Can you work these out from the model? Positions are in its coordinate system, mm. A direction names the side the tool comes from. Round coordinates to 2 decimals unless told otherwise and drop trailing zeros. Order: outer loops, then holes, each group sorted by start corner. A loop starts at its lowest first (then second) coordinate and runs counter-clockwise, first axis right, second up. Notation, with made-up numbers: (-25.75, -7.75) -> (26.25, -7.75) arc R19 cw to (26.25, -1.75) -> close; hole circle Ø5 at (52, 70.25). An arc over 180 degrees is marked (long way). Use a Markdown table: item, result. Add a question column.
Q1. If we section it at C-C on x = 32: List the corners of the cut face in (y, z) for me.
Q2. If we section it at D-D on y = -12: List the corners of the cut face in (x, z) for me.
Q3. I need wall thicknesses on line 1 along Y through (x, z) = (-16, 3.75); line 2 along X through (y, z) = (-30.5, 5.75); line 3 along Y through (x, z) = (-30.5, 6.75). Which ranges of each line are inside material? Lowest first, please. Write a range as [from, to].
Q4. If we section it at A-A on y = 0: List the corners of the cut face in (x, z) for me, plus the area to 3 significant figures.
Q5. I'm going to push flat-ended pins straight in: pin 1 Ø2.5 at (x, y) = (31.75, -31.75) entering from +Z; pin 2 Ø5 at (x, y) = (-35.5, 34) entering from +Z; pin 3 Ø3 at (x, z) = (-3.5, 2) entering from -Y; pin 4 Ø4 at (x, y) = (31.75, 31.75) entering from -Z. Where does each tip first touch, or does it pass through?
Q6. We'd pull the mould along Z, two halves only. Please class faces 1 (the face through (-12.07, 48.81, 3.7)), 2 (the face through (-23.629, 37.548, -0.887)), 3 (the face through (3.62, 37.87, 1.55)): +Z half, -Z half, draft (parallel to the pull), parting line (faces both ways), or undercut.
Q7. For faces 4 (the face through (11.986, 49.099, 3.698)), 5 (the face through (-10.254, -39.594, 3.698)), 6 (the face through (0, 50.1, 4)), which set-ups out of +Z, -Z, +X, -X, +Y, -Y let a thin tool reach every point of the face, with its end or its side?
Q8. If we section it at B-B on x = 0: List the corners of the cut face in (y, z) for me.
```python
from build123d import *

# Parameters (mm, degrees)
SKETCH_1_R               = 40.9
SKETCH_1_R_2             = 1.525
EXTRUDE_1_DEPTH          = 1.5
EXTRUDE_START            = -1.5
EXTRUDE_2_DEPTH          = 1.5
SKETCH_3_R               = 1.525
CUT_EXTRUDE_1_DEPTH      = 10
SKETCH_4_R               = 1.525
SKETCH_4_R_2             = 40.9
EXTRUDE_3_DEPTH          = 6
CUT_EXTRUDE_2_DEPTH      = 70.787248119
CUT_EXTRUDE_2_DEPTH_BACK = 70.787248119
EXTRUDE_4_DEPTH          = 2.5
EXTRUDE_5_REACH          = 106.028
EXTRUDE_5_END_RADIUS     = 48
SKETCH_9_R               = 1
CUT_EXTRUDE_3_DEPTH      = 105.027800787
CHAMFER_1_SIZE           = 1.2
CHAMFER_1_SIZE_2         = 2.827022839
CHAMFER_2_SIZE           = 1.091910703
CHAMFER_2_SIZE_2         = 3


with BuildPart() as part:
    # 草图1 → 凸台-拉伸1 (new body)
    with BuildSketch(Plane.XY):
        with BuildLine():
            Line((-12, 50.1), (12, 50.1))
            ThreePointArc((12, 50.1), (11.98646104, 49.112770637), (11.945854344, 48.126283833))
            ThreePointArc((11.945854344, 48.126283833), (12.311228539, 46.859989672), (13.385132402, 46.095967617))
            ThreePointArc((13.385132402, 46.095967617), (0.147817484, -47.999772395), (-13.668785094, 46.012653847))
            ThreePointArc((-13.668785094, 46.012653847), (-12.775478285, 46.565992731), (-12.285981368, 47.495817309))
            ThreePointArc((-12.285981368, 47.495817309), (-12.071709603, 48.790080839), (-12, 50.1))
        make_face()
        Circle(SKETCH_1_R, mode=Mode.SUBTRACT)
        with Locations((-17.153096541, 40.410163067)):
            Circle(SKETCH_1_R_2, mode=Mode.SUBTRACT)
        with Locations((12.835117837, 41.981778787)):
            Circle(SKETCH_1_R_2, mode=Mode.SUBTRACT)
    extrude(amount=EXTRUDE_1_DEPTH)

    # 草图2 → 凸台-拉伸2 (add)
    with BuildSketch(Plane.XY.offset(1.5).offset(EXTRUDE_START)):
        with BuildLine():
            Line((-19.201386918, 36.112556548), (-17.121235913, 32.200361501))
            ThreePointArc((-17.121235913, 32.200361501), (-16.264760822, 31.479428059), (-15.147630365, 31.55232629))
            ThreePointArc((-15.147630365, 31.55232629), (1.579071216, 34.964360914), (17.930115588, 30.058458959))
            ThreePointArc((17.930115588, 30.058458959), (18.570370617, 29.852165239), (19.236402831, 29.946423874))
            Line((19.236402831, 29.946423874), (25.180554341, 32.229639823))
            ThreePointArc((25.180554341, 32.229639823), (3.564669878, 40.744363152), (-19.201386918, 36.112556548))
        make_face()
    extrude(amount=EXTRUDE_2_DEPTH)

    # 草图3 → 切除-拉伸1 (cut)
    with BuildSketch(Plane.XY.offset(1.5)):
        with Locations((-31.749094475, 31.749094475)):
            Circle(SKETCH_3_R)
        with Locations((31.749094475, 31.749094475)):
            Circle(SKETCH_3_R)
        with Locations((31.749094475, -31.749094475)):
            Circle(SKETCH_3_R)
        with Locations((-31.749094475, -31.749094475)):
            Circle(SKETCH_3_R)
    extrude(amount=-CUT_EXTRUDE_1_DEPTH, mode=Mode.SUBTRACT)

    # 草图4 → 凸台-拉伸3 (add)
    with BuildSketch(Plane.XY.offset(1.5)):
        with BuildLine():
            Line((12, 50.1), (-12, 50.1))
            ThreePointArc((-12, 50.1), (-12.071709603, 48.790080839), (-12.285981368, 47.495817309))
            ThreePointArc((-12.285981368, 47.495817309), (-12.775478285, 46.565992731), (-13.668785094, 46.012653847))
            ThreePointArc((-13.668785094, 46.012653847), (0.147817484, -47.999772395), (13.385132402, 46.095967617))
            ThreePointArc((13.385132402, 46.095967617), (12.311228539, 46.859989672), (11.945854344, 48.126283833))
            ThreePointArc((11.945854344, 48.126283833), (11.98646104, 49.112770637), (12, 50.1))
        make_face()
        with Locations((-31.749094475, -31.749094475)):
            Circle(SKETCH_4_R, mode=Mode.SUBTRACT)
        with Locations((31.749094475, -31.749094475)):
            Circle(SKETCH_4_R, mode=Mode.SUBTRACT)
        with Locations((31.749094475, 31.749094475)):
            Circle(SKETCH_4_R, mode=Mode.SUBTRACT)
        with Locations((12.835117837, 41.981778787)):
            Circle(SKETCH_4_R, mode=Mode.SUBTRACT)
        with Locations((-31.749094475, 31.749094475)):
            Circle(SKETCH_4_R, mode=Mode.SUBTRACT)
        with Locations((-17.153096541, 40.410163067)):
            Circle(SKETCH_4_R, mode=Mode.SUBTRACT)
        with Locations(Location((0, 0, 0), (0, 0, 118))):
            Circle(SKETCH_4_R_2, mode=Mode.SUBTRACT)
    extrude(amount=EXTRUDE_3_DEPTH)

    # 草图5 → 切除-拉伸2 (cut, two sides: drawn at the far end of the back side and taken through both)
    with BuildSketch(Plane.XY.offset(7.5).offset(-CUT_EXTRUDE_2_DEPTH_BACK)):
        with BuildLine():
            ThreePointArc((-33.864147525, 29.482698526), (-34.848632515, 31.695578705), (-33.941125497, 33.941125497))
            ThreePointArc((-33.941125497, 33.941125497), (-48, 0), (-33.941125497, -33.941125497))
            ThreePointArc((-33.941125497, -33.941125497), (-34.848632515, -31.695578705), (-33.864147525, -29.482698526))
            ThreePointArc((-33.864147525, -29.482698526), (-44.9, 0), (-33.864147525, 29.482698526))
        make_face()
        with BuildLine():
            ThreePointArc((-29.482698526, -33.864147525), (-31.695578705, -34.848632515), (-33.941125497, -33.941125497))
            ThreePointArc((-33.941125497, -33.941125497), (1.4e-08, -48), (33.941125517, -33.941125477))
            ThreePointArc((33.941125517, -33.941125477), (31.695578719, -34.848632516), (29.482698526, -33.864147525))
            ThreePointArc((29.482698526, -33.864147525), (0, -44.9), (-29.482698526, -33.864147525))
        make_face()
        with BuildLine():
            ThreePointArc((33.864147525, -29.482698526), (34.848632515, -31.695578691), (33.941125517, -33.941125477))
            ThreePointArc((33.941125517, -33.941125477), (48, 1.4e-08), (33.941125497, 33.941125497))
            ThreePointArc((33.941125497, 33.941125497), (34.848632515, 31.695578705), (33.864147525, 29.482698526))
            ThreePointArc((33.864147525, 29.482698526), (44.9, 0), (33.864147525, -29.482698526))
        make_face()
    extrude(amount=CUT_EXTRUDE_2_DEPTH + CUT_EXTRUDE_2_DEPTH_BACK, mode=Mode.SUBTRACT)

    # 草图6 → 凸台-拉伸4 (add)
    with BuildSketch(Plane(origin=(0, 0, 0), x_dir=(-1, 0, 0), z_dir=(0, 0, -1))):
        with BuildLine():
            Line((20, 35.676462829), (24.203821377, 32.969456027))
            ThreePointArc((24.203821377, 32.969456027), (22.14331564, 34.387258868), (20, 35.676462829))
        make_face()
    extrude(amount=-EXTRUDE_4_DEPTH)

    # 凸台-拉伸5: up to this cylinder (the profile starts inside it)
    extrude_5_end = Plane(origin=(0, 0, -1.061033), z_dir=(0, 0, -1)) * Cylinder(EXTRUDE_5_END_RADIUS, 309.056, mode=Mode.PRIVATE)
    # 草图8 → 凸台-拉伸5 (add, up to the surface)
    with BuildSketch(Plane(origin=(-22.101910689, 34.322959428, 0), x_dir=(0.8407642754995168, 0.5414013604007407, 0), z_dir=(0.5414013604007407, -0.8407642754995168, 0)), mode=Mode.PRIVATE) as extrude_5_sk1:
        with BuildLine():
            Line((-2.5, 0), (2.5, 0))
            ThreePointArc((2.5, 0), (0, -2.5), (-2.5, 0))
        make_face()
    extrude_5_tool1 = extrude(extrude_5_sk1.sketch, amount=-EXTRUDE_5_REACH, mode=Mode.PRIVATE) & extrude_5_end
    add(extrude_5_tool1.solids().sort_by_distance((-22.101911, 34.322959, -1.061033))[0])

    # 草图9 → 切除-拉伸3 (cut, through all)
    with BuildSketch(Plane(origin=(-22.101910689, 34.322959428, 0), x_dir=(0.8407642754995168, 0.5414013604007407, 0), z_dir=(0.5414013604007407, -0.8407642754995168, 0))):
        Circle(SKETCH_9_R)
    extrude(amount=-CUT_EXTRUDE_3_DEPTH, mode=Mode.SUBTRACT)

    # 倒角1
    # the kernel refuses this chamfer: 2.827022839, 1.2 mm, written as the material it takes off along each edge
    with BuildSketch(Plane(origin=(0, 0, 1.5), x_dir=(-0.6107495991650607, 0.79182379802562, 0), z_dir=(-0.79182379802562, -0.6107495991650607, 0))) as chamfer_1_piece_1:
        Polygon((35, CHAMFER_1_SIZE), (35 + CHAMFER_1_SIZE_2, 0), (35, 0), align=None)
    revolve(axis=Axis((0, 0, 1.5), (0, 0, -1)), revolution_arc=80.459152239, mode=Mode.SUBTRACT)

    # 倒角2
    # the kernel refuses this chamfer: 3, 1.091910703 mm, written as the material it adds along each edge
    with BuildSketch(Plane(origin=(0, 0, 1.5), x_dir=(0.7536182445133375, 0.6573123622271496, 0), z_dir=(0.6573123622271496, -0.7536182445133375, 0))) as chamfer_2_piece_1_section:
        Polygon((40.9, CHAMFER_2_SIZE), (40.9 - CHAMFER_2_SIZE_2, 0), (40.9, 0), align=None)
    chamfer_2_piece_1 = revolve(axis=Axis((0, 0, 1.5), (0, 0, 1)), revolution_arc=76.90478106, mode=Mode.PRIVATE)
    chamfer_2_piece_1 = split(chamfer_2_piece_1, bisect_by=Plane(origin=(8.613354957, 25.865990815, 2.004229424), z_dir=(-0.35856914515570787, 0.933503169861948, 0)), keep=Keep.TOP, mode=Mode.PRIVATE)
    add(chamfer_2_piece_1)


solid = part.part
```
Answer below:
| question | item | result |
|---|---|---|
| 1 | outline | (-34.84, 0) -> (-33.25, 0) -> (-33.25, 7.5) -> (-34.84, 7.5) -> close; (-30.24, 0) -> (-25.47, 0) -> (-25.47, 7.5) -> (-30.24, 7.5) -> close; (25.47, 0) -> (30.24, 0) -> (30.24, 7.5) -> (25.47, 7.5) -> close; (33.25, 0) -> (35.78, 0) -> (35.78, 7.5) -> (33.25, 7.5) -> close |
| 2 | outline | (-43.27, 0) -> (-39.1, 0) -> (-39.1, 7.5) -> (-43.27, 7.5) -> close; (39.1, 0) -> (43.27, 0) -> (43.27, 7.5) -> (39.1, 7.5) -> close |
| 3 | line 1 | [-41.95, -37.64], [37.64, 39.41], [41.41, 45.25] |
| 3 | line 2 | [-34.59, -32.62], [-30.87, -27.25], [27.25, 30.87], [32.62, 34.59] |
| 3 | line 3 | [-34.59, -32.62], [-30.87, -27.25], [27.25, 30.87], [32.62, 37.06] |
| 4 | outline | (-44.9, 0) -> (-40.9, 0) -> (-40.9, 7.5) -> (-44.9, 7.5) -> close; (40.9, 0) -> (44.9, 0) -> (44.9, 7.5) -> (40.9, 7.5) -> close |
| 4 | area | 60.0 mm² |
| 5 | pin 1 | through |
| 5 | pin 2 | z = 7.5 |
| 5 | pin 3 | y = -44.86 |
| 5 | pin 4 | z = 0 |
| 6 | face 1 | draft |
| 6 | face 2 | undercut |
| 6 | face 3 | +Z half |
| 7 | face 4 | +Z, -Z, +X |
| 7 | face 5 | +Z |
| 7 | face 6 | +Z, -Z, +X, -X, +Y |
| 8 | outline | (-44.9, 0) -> (-40.9, 0) -> (-40.9, 7.5) -> (-44.9, 7.5) -> close; (35, 0) -> (50.1, 0) -> (50.1, 7.5) -> (40.9, 7.5) -> (40.9, 2.59) -> (37.9, 1.5) -> (37.83, 1.5) -> (35, 0.3) -> close |
